```python
from build123d import *

# Parameters (mm, degrees)
F0_R     = 3.1
F1_DEPTH = 10
F3_DEPTH = 5
F4_R     = 1.1706515684
F5_DEPTH = 25


with BuildPart() as f1:
    # F0 (on Right) → F1 (new body)
    with BuildSketch(Plane.YZ):
        Circle(F0_R)
    extrude(amount=F1_DEPTH)

    # F2 (on face) → F3 (join)
    with BuildSketch(Plane.YZ.offset(10)):
        with BuildLine():
            ThreePointArc((3.1, -11.2293484316), (6.3047601065, -8.4620192023), (7.5, -4.4))
            ThreePointArc((7.5, -4.4), (6.3047601065, -0.3379807977), (3.1, 2.4293484316))
            Line((3.1, 2.4293484316), (3.1, -11.2293484316))
        make_face()
        with BuildLine():
            Line((-3.1, 2.4293484316), (3.1, 2.4293484316))
            ThreePointArc((3.1, 2.4293484316), (0, 3.1), (-3.1, 2.4293484316))
        make_face()
        with BuildLine():
            Line((3.1, -11.2293484316), (3.1, 2.4293484316))
            Line((3.1, 2.4293484316), (-3.1, 2.4293484316))
            Line((-3.1, 2.4293484316), (-3.1, -11.2293484316))
            ThreePointArc((-3.1, -11.2293484316), (0, -11.9), (3.1, -11.2293484316))
        make_face()
        with BuildLine():
            Line((3.1, -13.5706515684), (3.1, -11.2293484316))
            ThreePointArc((3.1, -11.2293484316), (0, -11.9), (-3.1, -11.2293484316))
            Line((-3.1, -11.2293484316), (-3.1, -13.5706515684))
            Line((-3.1, -13.5706515684), (3.1, -13.5706515684))
        make_face()
        with BuildLine():
            Line((-3.1, -11.2293484316), (-3.1, 2.4293484316))
            ThreePointArc((-3.1, 2.4293484316), (-7.5, -4.4), (-3.1, -11.2293484316))
        make_face()
    extrude(amount=F3_DEPTH)

    # F4 (on face) → F5 (join)
    with BuildSketch(Plane.XZ.offset(3.1)):
        with Locations((12.5, -12.4)):
            Circle(F4_R)
    extrude(amount=F5_DEPTH)

    # F6: F1 across face


with BuildPart() as f1_1:
    add(f1.part)
    add(f1.part.mirror(Plane(origin=(0, 0, 0), x_dir=(0, 1, 0), z_dir=(-1, 0, 0))))


solid = f1_1.part
```
Geometry: final body of the model. Coordinates: model frame, mm. A direction names the side the tool comes from. Round coordinates to 2 decimals unless told otherwise and drop trailing zeros. Order: outer loops, then holes, each group sorted by start corner. A loop starts at its lowest first (then second) coordinate and runs counter-clockwise, first axis right, second up. Notation, with made-up numbers: (32, 44) -> (36, 44) arc R5 ccw to (36, 50) -> close; hole circle Ø9 at (-6.5, 33.5). An arc over 180 degrees is marked (long way). Write each question's results on one line, items separated by ' | '.
Q1. Section query B-B (y = -24.5). Output: boundary loops of the cut face in (x, z).
Response values:
outline: circle Ø2.34 at (-12.5, -12.4); circle Ø2.34 at (12.5, -12.4)
Q2. Pin query (flat end, axial travel): pin 1 Ø2 at (x, z) = (-11, -3) entering from +Y; pin 2 Ø2.5 at (x, z) = (-11.5, -12) entering from +Y; pin 3 Ø1.5 at (x, y) = (2.5, 2) entering from -Z. Return the tip coordinate at first contact, or that it passes through.
Response values:
pin 1: y = 7.49 | pin 2: y = 3.99 | pin 3: z = -2.84
Q3. Section query A-A (z = -12.4). Output: boundary loops of the cut face in (x, y), and give its area (3 significant figures).
Response values:
outline: (-15, -3.1) -> (-13.67, -3.1) -> (-13.67, -28.1) -> (-11.33, -28.1) -> (-11.33, -3.1) -> (-10, -3.1) -> (-10, 3.1) -> (-15, 3.1) -> close; (10, -3.1) -> (11.33, -3.1) -> (11.33, -28.1) -> (13.67, -28.1) -> (13.67, -3.1) -> (15, -3.1) -> (15, 3.1) -> (10, 3.1) -> close | area: 179 mm²
Q4. Ray query, line 1 along X through (y, z) = (6.5, -2.25); line 2 along Z through (x, y) = (8, -0.5); line 3 along Z through (x, y) = (13.5, -21.5). Return the intervals inside material, ascending.
Response values:
line 1: -15 to -10, 10 to 15 | line 2: -3.06 to 3.06 | line 3: -13.01 to -11.79
Q5. Section query C-C (z = -2.5). Output: boundary loops of the cut face in (x, y).
Response values:
outline: (-15, -7.26) -> (-10, -7.26) -> (-10, -1.83) -> (10, -1.83) -> (10, -7.26) -> (15, -7.26) -> (15, 7.26) -> (10, 7.26) -> (10, 1.83) -> (-10, 1.83) -> (-10, 7.26) -> (-15, 7.26) -> close
Q6. Access query for faces 1 (the face through (-12, 0, -13.571)), 2 (the face through (13.04, -15.42, -13.44)), 3 (the face through (-12, 3.1, -12)). Directions: +Z, -Z, +X, -X, +Y, -Y. A direction counts if a zero-diameter tool reaches every point of the face in a straight line with its end or side. Return the directions, or none.
Response values:
face 1: -Z, +X, -X, +Y, -Y | face 2: -Y | face 3: -Z, +X, -X, +Y
Q7. Section query D-D (z = -8.25). Output: boundary loops of the cut face in (x, y), and give its area (3 significant figures).
Response values:
outline: (-15, -6.44) -> (-10, -6.44) -> (-10, 6.44) -> (-15, 6.44) -> close; (10, -6.44) -> (15, -6.44) -> (15, 6.44) -> (10, 6.44) -> close | area: 129 mm²
